Geometry: final body of the model. Coordinates: model frame, mm. A direction names the side the tool comes from. Give positions to 0.01 mm unless a question says otherwise; leave off trailing zeros. Order: outer loops, then holes, each group sorted by start corner. A loop starts at its lowest first (then second) coordinate and runs counter-clockwise, first axis right, second up. Notation, with made-up numbers: (56.5, 74.25) - (64.5, 74.25) arc R27 cw to (64.5, 103.25) - close; hole circle Ø5 at (-12, 67). An arc over 180 degrees is marked (long way). Put each result on its own line as item: value. Start each with the question number.
1. Mould query, pull axis X, two halves, no side actions, for faces 1 (the cylindrical face through (-17.36, 80.14, 20.4)), 2 (the cylindrical face through (17.36, 97.54, -14.4)), 3 (the cylindrical face through (-17.914, 4.31, -16.708)), 4 (the flat face through (-21, 8.5, -18)). Classes: pulls with the +X half, pulls with the -X half, needs draft (parallel to the pull), parting line crosses it, or undercut.
2. Section B-B on y = 63.5. Count the separate pieces of the cut face and the enclosed holes in it, plus the area to 3 significant figures.
3. Section A-A on z = -0.5. Return the cut outline in (x, y).
4. Ray query, line 1 along X through (y, z) = (59.5, 22.5); line 2 along X through (y, z) = (49.5, -2); line 3 along Y through (x, z) = (18.5, 21). Return the intervals inside material, ascending. Write a range as from..to.
5. First-contact query: P1, Ø1.9, axis at x = -19.5, z = -16.5, coming from the +Y side; P2, Ø0.9, axis at x = 21.5, y = 98.5, coming from the +Z side; P3, Ø2.5, axis at x = -21, y = 96.5, coming from the -Z side; P4, Ø5, axis at x = -19.5, z = 22.5, coming from the +Y side. Flat tips, straight axial feed; report the tip coordinate or a pass-through.
6. Set-up query: faces 5 (the flat face through (-21, 98, 19.5)), 6 (the flat face through (-9, 51, 0)), 7 (the flat face through (-21, 90, -18)), 8 (the flat face through (-21, 70, 24)). Return all of +Z, -Z, +X, -X, +Y, -Y with unobstructed straight access to the full face (end or side cutting, diameter ignored); none if empty.
from build123d import *

# Parameters (mm, degrees)
SKETCH_1_W          = 45
SKETCH_1_H          = 39
SKETCH_1_R          = 12.5
EXTRUDE_1_DEPTH     = 100
SKETCH_2_W          = 6
SKETCH_2_H          = 6
EXTRUDE_2_DEPTH     = 100
SKETCH_3_W          = 45
SKETCH_3_H          = 100
EXTRUDE_3_DEPTH     = 6
SKETCH_4_R          = 1.6
CUT_EXTRUDE_1_DEPTH = 106.624334317
CUT_EXTRUDE_2_DEPTH = 5
CUT_EXTRUDE_4_DEPTH = 20
SKETCH_9_W          = 6.3
SKETCH_9_H          = 6.3
CUT_EXTRUDE_5_DEPTH = 95
CUT_EXTRUDE_START   = -20
CUT_EXTRUDE_6_DEPTH = 20
CHAMFER_1_SIZE      = 1
CHAMFER_2_SIZE      = 0.5
CHAMFER_3_SIZE      = 0.5
CHAMFER_4_SIZE      = 3.5


with BuildPart() as part:
    # 草图1 → 凸台-拉伸1 (new body)
    with BuildSketch(Plane(origin=(0, 0, 0), x_dir=(1, 0, 0), z_dir=(0, 1, 0))):
        Rectangle(SKETCH_1_W, SKETCH_1_H)
        with Locations(Location((0, 0, 0), (0, 0, 270))):
            Circle(SKETCH_1_R, mode=Mode.SUBTRACT)
    extrude(amount=EXTRUDE_1_DEPTH)

    # 草图2 → 凸台-拉伸2 (add)
    with BuildSketch(Plane(origin=(0, 100, 0), x_dir=(1, 0, 0), z_dir=(0, 1, 0))):
        with Locations((12, 0)):
            Rectangle(SKETCH_2_W, SKETCH_2_H)
        with Locations((-12, 0)):
            Rectangle(SKETCH_2_W, SKETCH_2_H)
    extrude(amount=-EXTRUDE_2_DEPTH)

    # 草图3 → 凸台-拉伸3 (add)
    with BuildSketch(Plane.XY.offset(19.5)):
        with Locations((0, 50)):
            Rectangle(SKETCH_3_W, SKETCH_3_H)
    extrude(amount=EXTRUDE_3_DEPTH)

    # 草图4 → 切除-拉伸1 (cut, through all)
    with BuildSketch(Plane(origin=(0, 100, 0), x_dir=(1, 0, 0), z_dir=(0, 1, 0))):
        with Locations(Location((-19.5, 16.5, 0), (0, 0, 270))):
            Circle(SKETCH_4_R)
        with Locations(Location((19.5, 16.5, 0), (0, 0, 90))):
            Circle(SKETCH_4_R)
        with Locations(Location((19.5, -22.5, 0), (0, 0, 270))):
            Circle(SKETCH_4_R)
        with Locations(Location((-19.5, -22.5, 0), (0, 0, 90))):
            Circle(SKETCH_4_R)
    extrude(amount=-CUT_EXTRUDE_1_DEPTH, mode=Mode.SUBTRACT)

    # 草图5 → 切除-拉伸2 (cut)
    with BuildSketch(Plane(origin=(0, 100, 0), x_dir=(1, 0, 0), z_dir=(0, 1, 0))):
        with BuildLine():
            Line((-19.5, 13.5), (-22.5, 13.5))
            Line((-22.5, 13.5), (-22.5, 19.5))
            Line((-22.5, 19.5), (-16.5, 19.5))
            Line((-16.5, 19.5), (-16.5, 16.5))
            ThreePointArc((-16.5, 16.5), (-17.378679656, 14.378679656), (-19.5, 13.5))
        make_face()
        with BuildLine():
            Line((22.5, 19.5), (16.5, 19.5))
            Line((16.5, 19.5), (16.5, 16.5))
            ThreePointArc((16.5, 16.5), (17.378679656, 14.378679656), (19.5, 13.5))
            Line((19.5, 13.5), (22.5, 13.5))
            Line((22.5, 13.5), (22.5, 19.5))
        make_face()
        with BuildLine():
            Line((22.5, -19.5), (22.5, -25.5))
            Line((22.5, -25.5), (16.5, -25.5))
            Line((16.5, -25.5), (16.5, -22.5))
            ThreePointArc((16.5, -22.5), (17.378679656, -20.378679656), (19.5, -19.5))
            Line((19.5, -19.5), (22.5, -19.5))
        make_face()
        with BuildLine():
            Line((-22.5, -25.5), (-16.5, -25.5))
            Line((-16.5, -25.5), (-16.5, -22.5))
            ThreePointArc((-16.5, -22.5), (-17.378679656, -20.378679656), (-19.5, -19.5))
            Line((-19.5, -19.5), (-22.5, -19.5))
            Line((-22.5, -19.5), (-22.5, -25.5))
        make_face()
    extrude(amount=-CUT_EXTRUDE_2_DEPTH, mode=Mode.SUBTRACT)

    # 草图8 → 切除-拉伸4 (cut)
    with BuildSketch(Plane(origin=(0, 90, 0), x_dir=(1, 0, 0), z_dir=(0, 1, 0))):
        with BuildLine():
            Line((-22.5, 13.5), (-19.5, 13.5))
            ThreePointArc((-19.5, 13.5), (-17.378679656, 14.378679656), (-16.5, 16.5))
            Line((-16.5, 16.5), (-16.5, 19.5))
            Line((-16.5, 19.5), (-22.5, 19.5))
            Line((-22.5, 19.5), (-22.5, 13.5))
        make_face()
        with BuildLine():
            Line((22.5, 19.5), (16.5, 19.5))
            Line((16.5, 19.5), (16.5, 16.5))
            ThreePointArc((16.5, 16.5), (17.378679656, 14.378679656), (19.5, 13.5))
            Line((19.5, 13.5), (22.5, 13.5))
            Line((22.5, 13.5), (22.5, 19.5))
        make_face()
        with BuildLine():
            Line((-22.5, -25.5), (-16.5, -25.5))
            Line((-16.5, -25.5), (-16.5, -22.5))
            ThreePointArc((-16.5, -22.5), (-17.378679656, -20.378679656), (-19.5, -19.5))
            Line((-19.5, -19.5), (-22.5, -19.5))
            Line((-22.5, -19.5), (-22.5, -25.5))
        make_face()
        with BuildLine():
            Line((16.5, -22.5), (16.5, -25.5))
            Line((16.5, -25.5), (22.5, -25.5))
            Line((22.5, -25.5), (22.5, -19.5))
            Line((22.5, -19.5), (19.5, -19.5))
            ThreePointArc((19.5, -19.5), (17.378679656, -20.378679656), (16.5, -22.5))
        make_face()
    extrude(amount=-CUT_EXTRUDE_4_DEPTH, mode=Mode.SUBTRACT)

    # 草图9 → 切除-拉伸5 (cut)
    with BuildSketch(Plane.XZ):
        with Locations((0, 12)):
            Rectangle(SKETCH_9_W, SKETCH_9_H)
        with Locations((0, -12)):
            Rectangle(SKETCH_9_W, SKETCH_9_H)
    extrude(amount=-CUT_EXTRUDE_5_DEPTH, mode=Mode.SUBTRACT)

    # 草图10 → 切除-拉伸6 (cut)
    with BuildSketch(Plane(origin=(0, 8.5, 0), x_dir=(-1, 0, 0), z_dir=(0, -1, 0)).offset(CUT_EXTRUDE_START)):
        with BuildLine():
            Line((-16.5, 19.5), (-22.5, 19.5))
            Line((-22.5, 19.5), (-22.5, 13.5))
            Line((-22.5, 13.5), (-19.5, 13.5))
            ThreePointArc((-19.5, 13.5), (-17.378679656, 14.378679656), (-16.5, 16.5))
            Line((-16.5, 16.5), (-16.5, 19.5))
        make_face()
        with BuildLine():
            Line((19.5, 13.5), (22.5, 13.5))
            Line((22.5, 13.5), (22.5, 19.5))
            Line((22.5, 19.5), (16.5, 19.5))
            Line((16.5, 19.5), (16.5, 16.5))
            ThreePointArc((16.5, 16.5), (17.378679656, 14.378679656), (19.5, 13.5))
        make_face()
        with BuildLine():
            Line((-16.5, -25.5), (-16.5, -22.5))
            ThreePointArc((-16.5, -22.5), (-17.378679656, -20.378679656), (-19.5, -19.5))
            Line((-19.5, -19.5), (-22.5, -19.5))
            Line((-22.5, -19.5), (-22.5, -25.5))
            Line((-22.5, -25.5), (-16.5, -25.5))
        make_face()
        with BuildLine():
            Line((22.5, -19.5), (19.5, -19.5))
            ThreePointArc((19.5, -19.5), (17.378679656, -20.378679656), (16.5, -22.5))
            Line((16.5, -22.5), (16.5, -25.5))
            Line((16.5, -25.5), (22.5, -25.5))
            Line((22.5, -25.5), (22.5, -19.5))
        make_face()
    extrude(amount=CUT_EXTRUDE_6_DEPTH, mode=Mode.SUBTRACT)

    # 倒角1
    chamfer_1_edges = [part.edges().sort_by_distance(p)[0] for p in [
        (-22.5, 92.5, -19.5),
        (22.5, 92.5, -19.5),
        (-22.5, 49.25, 25.5),
        (22.5, 92.5, 25.5),
        (-22.5, 49.25, -19.5),
        (22.5, 49.25, -19.5),
        (-22.5, 4.25, 25.5),
        (22.5, 49.25, 25.5),
        (-22.5, 4.25, -19.5),
        (22.5, 4.25, -19.5),
        (22.5, 4.25, 25.5),
        (-22.5, 92.5, 25.5),
    ]]
    chamfer(chamfer_1_edges, length=CHAMFER_1_SIZE)

    # 倒角2
    chamfer_2_edges = [part.edges().sort_by_distance(p)[0] for p in [
        (0, 100, -12.5),
        (8.893379874, 0, -8.783950957),
        (10.56733055, 100, 3),
        (10.56733055, 100, -3),
        (9, 100, 0),
        (10.56733055, 0, 3),
        (8.893379874, 0, 8.783950957),
        (9, 0, 0),
        (-8.893379874, 0, -8.783950957),
        (-3.15, 0, -13.623295214),
        (10.56733055, 0, -3),
        (3.15, 0, 13.623295214),
        (0, 0, 15.15),
        (-3.15, 0, 13.623295214),
        (3.15, 0, -13.623295214),
        (0, 0, -15.15),
        (-8.893379874, 0, 8.783950957),
        (0, 100, 12.5),
        (-10.56733055, 100, 3),
        (-9, 100, 0),
        (-10.56733055, 100, -3),
        (-10.56733055, 0, -3),
        (-9, 0, 0),
        (-10.56733055, 0, 3),
    ]]
    chamfer(chamfer_2_edges, length=CHAMFER_2_SIZE)

    # 倒角3
    chamfer_3_edges = [part.edges().sort_by_distance(p)[0] for p in [
        (9, 50, -3),
        (9, 50, 3),
        (-9, 50, 3),
        (-9, 50, -3),
    ]]
    chamfer(chamfer_3_edges, length=CHAMFER_3_SIZE)

    # 倒角4
    # the kernel refuses this chamfer: 3.5 mm, written as the material it takes off along each edge
    with BuildSketch(Plane(origin=(0, 95, 0), x_dir=(0.8276166143248335, 0, 0.5612938087076144), z_dir=(0.5612938087076144, 0, -0.8276166143248335))) as chamfer_4_piece_1_section:
        Polygon((12.5, -CHAMFER_4_SIZE), (12.5 + CHAMFER_4_SIZE, 0), (12.5, 0), align=None)
    chamfer_4_piece_1 = revolve(axis=Axis((0, 95, 0), (0, -1, 0)), revolution_arc=111.709358924, mode=Mode.PRIVATE)
    chamfer_4_piece_1 = split(chamfer_4_piece_1, bisect_by=Plane(origin=(3.15, 96.215607444, 13.411571033), z_dir=(-1, 0, 0)), keep=Keep.TOP, mode=Mode.PRIVATE)
    chamfer_4_piece_1 = split(chamfer_4_piece_1, bisect_by=Plane(origin=(0, 96.215607444, 15.15), z_dir=(0, 0, -1)), keep=Keep.TOP, mode=Mode.PRIVATE)
    chamfer_4_piece_1 = split(chamfer_4_piece_1, bisect_by=Plane(origin=(-3.15, 96.215607444, 13.411571033), z_dir=(1, 0, 0)), keep=Keep.TOP, mode=Mode.PRIVATE)
    add(chamfer_4_piece_1, mode=Mode.SUBTRACT)
    with BuildSketch(Plane(origin=(0, 95, 0), x_dir=(-0.8276166143248334, 0, -0.5612938087076144), z_dir=(-0.5612938087076144, 0, 0.8276166143248334))) as chamfer_4_piece_2_section:
        Polygon((12.5, -CHAMFER_4_SIZE), (12.5 + CHAMFER_4_SIZE, 0), (12.5, 0), align=None)
    chamfer_4_piece_2 = revolve(axis=Axis((0, 95, 0), (0, -1, 0)), revolution_arc=111.709358924, mode=Mode.PRIVATE)
    chamfer_4_piece_2 = split(chamfer_4_piece_2, bisect_by=Plane(origin=(3.15, 96.215607444, -13.411571033), z_dir=(-1, 0, 0)), keep=Keep.TOP, mode=Mode.PRIVATE)
    chamfer_4_piece_2 = split(chamfer_4_piece_2, bisect_by=Plane(origin=(0, 96.215607444, -15.15), z_dir=(0, 0, 1)), keep=Keep.TOP, mode=Mode.PRIVATE)
    chamfer_4_piece_2 = split(chamfer_4_piece_2, bisect_by=Plane(origin=(-3.15, 96.215607444, -13.411571033), z_dir=(1, 0, 0)), keep=Keep.TOP, mode=Mode.PRIVATE)
    add(chamfer_4_piece_2, mode=Mode.SUBTRACT)


solid = part.part
Resolved:
1. face 1: pulls with the -X half
1. face 2: pulls with the +X half
1. face 3: undercut
1. face 4: needs draft
2. separate pieces: 1
2. enclosed holes: 5
2. area: 1,500 mm^2
3. outline: (-22.5, 0) - (-9.5, 0) - (-9, 0.5) - (-9, 99.5) - (-9.5, 100) - (-22.5, 100) - close; (9, 0.5) - (9.5, 0) - (22.5, 0) - (22.5, 100) - (9.5, 100) - (9, 99.5) - close
4. line 1: -22.5..-21.1, -17.9..17.9, 21.1..22.5
4. line 2: -22.5..-9, 9..22.5
4. line 3: 0..8.5, 28.5..70, 90..95
5. P1: through
5. P2: z = 19.5
5. P3: z = -13.5
5. P4: y = 95
6. face 5: +Z, -X, +Y
6. face 6: +Y, -Y
6. face 7: -Z, -X
6. face 8: +Z, -X
